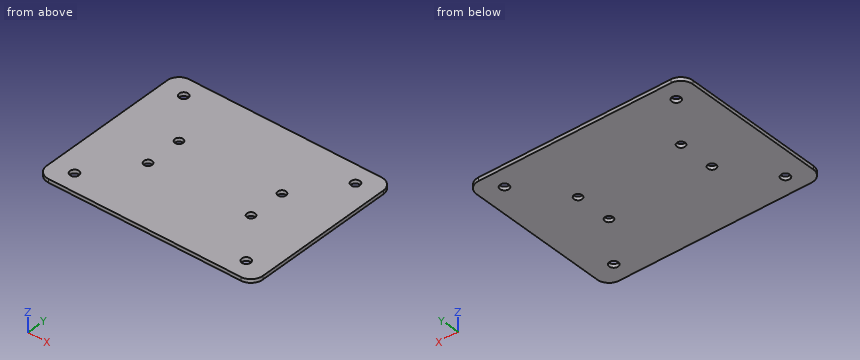
from build123d import *

# Parameters (mm, degrees)
SKETCH1_W           = 73
SKETCH1_H           = 56
SKETCH1_R           = 1.5
BOSS_EXTRUDE1_DEPTH = 1.2
FILLET1_R           = 4
CUT_EXTRUDE1_REACH  = 94.013
SKETCH2_R           = 1.375


with BuildPart() as part:
    # Sketch1 → Boss-Extrude1 (new body)
    with BuildSketch(Plane.XY):
        with Locations((36.5, 28)):
            Rectangle(SKETCH1_W, SKETCH1_H)
        with Locations((7.5, 6.25)):
            Circle(SKETCH1_R, mode=Mode.SUBTRACT)
        with Locations(Location((65.5, 6.25, 0), (0, 0, 180))):
            Circle(SKETCH1_R, mode=Mode.SUBTRACT)
        with Locations((65.5, 49.75)):
            Circle(SKETCH1_R, mode=Mode.SUBTRACT)
        with Locations(Location((7.5, 49.75, 0), (0, 0, 180))):
            Circle(SKETCH1_R, mode=Mode.SUBTRACT)
    extrude(amount=BOSS_EXTRUDE1_DEPTH)

    # Fillet1
    fillet1_edges = [part.edges().sort_by_distance(p)[0] for p in [
        (0, 56, 0.6),
        (73, 56, 0.6),
        (73, 0, 0.6),
        (0, 0, 0.6),
    ]]
    fillet(fillet1_edges, radius=FILLET1_R)

    # Sketch2 → Cut-Extrude1 (cut, up to next)
    with BuildSketch(Plane.XY.offset(1.2), mode=Mode.PRIVATE) as cut_extrude1_sk1:
        with Locations((53.89, 21.84)):
            Circle(SKETCH2_R)
    cut_extrude1_tool1 = extrude(cut_extrude1_sk1.sketch, amount=-CUT_EXTRUDE1_REACH, mode=Mode.PRIVATE) & part.part
    # Sketch2 → Cut-Extrude1 (cut, up to next)
    with BuildSketch(Plane.XY.offset(1.2), mode=Mode.PRIVATE) as cut_extrude1_sk2:
        with Locations(Location((53.89, 34.16, 0), (0, 0, 180))):
            Circle(SKETCH2_R)
    cut_extrude1_tool2 = extrude(cut_extrude1_sk2.sketch, amount=-CUT_EXTRUDE1_REACH, mode=Mode.PRIVATE) & part.part
    # Sketch2 → Cut-Extrude1 (cut, up to next)
    with BuildSketch(Plane.XY.offset(1.2), mode=Mode.PRIVATE) as cut_extrude1_sk3:
        with Locations(Location((19.11, 21.84, 0), (0, 0, 180))):
            Circle(SKETCH2_R)
    cut_extrude1_tool3 = extrude(cut_extrude1_sk3.sketch, amount=-CUT_EXTRUDE1_REACH, mode=Mode.PRIVATE) & part.part
    # Sketch2 → Cut-Extrude1 (cut, up to next)
    with BuildSketch(Plane.XY.offset(1.2), mode=Mode.PRIVATE) as cut_extrude1_sk4:
        with Locations((19.11, 34.16)):
            Circle(SKETCH2_R)
    cut_extrude1_tool4 = extrude(cut_extrude1_sk4.sketch, amount=-CUT_EXTRUDE1_REACH, mode=Mode.PRIVATE) & part.part
    add(cut_extrude1_tool1.solids().sort_by_distance((53.89, 21.84, 1.2))[0], mode=Mode.SUBTRACT)
    add(cut_extrude1_tool2.solids().sort_by_distance((53.89, 34.16, 1.2))[0], mode=Mode.SUBTRACT)
    add(cut_extrude1_tool3.solids().sort_by_distance((19.11, 21.84, 1.2))[0], mode=Mode.SUBTRACT)
    add(cut_extrude1_tool4.solids().sort_by_distance((19.11, 34.16, 1.2))[0], mode=Mode.SUBTRACT)


solid = part.part
Verification items for the finished model (mm, model axes). Coordinates: 2 decimals unless noted, no trailing zeros. Loops run counter-clockwise (first coordinate to the right, second up) from the corner with the lowest first, then second, coordinate; pieces in that order, holes last. Notation, with made-up numbers: M 72,44.5 L 107,44.5 A26 cw 107,72.5 Z; hole C -36,12.25 d10. An arc over 180 degrees is marked long. One line per item, written item: value.
1. Section check C-C on z = 0.7. Give the number of separate pieces and of enclosed holes in the cut face, plus the area to 3 significant figures.
Answers follow:
separate pieces: 1
enclosed holes: 8
area: 4,020 mm^2
2. Section check B-B on x = 7.5. Record the cut outline in (y, z), plus the area to 3 significant figures.
Answers follow:
outline: M 0,0 L 4.75,0 L 4.75,1.2 L 0,1.2 Z; M 7.75,0 L 48.25,0 L 48.25,1.2 L 7.75,1.2 Z; M 51.25,0 L 56,0 L 56,1.2 L 51.25,1.2 Z
area: 60.0 mm^2
3. Section check A-A on y = 34.16. Record the cut outline in (x, z) (3 decimals).
Answers follow:
outline: M 0,0 L 17.735,0 L 17.735,1.2 L 0,1.2 Z; M 20.485,0 L 52.515,0 L 52.515,1.2 L 20.485,1.2 Z; M 55.265,0 L 73,0 L 73,1.2 L 55.265,1.2 Z
4. Material ranges on line 1 along Y through (x, z) = (7.5, 0.6); line 2 along Y through (x, z) = (19.11, 0.6) (3 decimals), recorded low to high. Write a range as from..to.
Answers follow:
line 1: 0..4.75, 7.75..48.25, 51.25..56
line 2: 0..20.465, 23.215..32.785, 35.535..56
5. Gauge pin test, flat end, axial feed: P1, Ø2.5, axis at x = 65.5, y = 6.25, coming from the -Z side. Record the tip position at first contact, or that the pin passes through.
Answers follow:
P1: through
